Model file for the job. Use its own axes, mm. Coordinates: 2 decimals unless noted, no trailing zeros. Use CSV: the item, a comma, the result in double quotes. Start each with the question number.
(1) Cut at A-A on y = 1.25. Give the number of separate pieces and of enclosed holes in the cut face, plus the area to 3 significant figures.
(2) Probe L1, parallel to X at y = 1.95, z = 139.7; L2, parallel to X at y = 2.3, z = 19 (3 decimals); L3, parallel to Z at x = 38.5, y = 1.1. List the from-to ranges inside material, lowest first.
(3) Pin check, flat tip, straight feed: pin 1 Ø3 at (x, z) = (21.01, -39.81) entering from +Y. Stop position of the tip, or through.
```python
from build123d import *

# Parameters (mm, degrees)
PLATE_THICKNESS_DEPTH        = 3.175
SKETCH3_R                    = 2.159
MOUNTING_HOLES_DEPTH         = 159.781746826
SKETCH4_R                    = 1.905
JETSON_HOLES_W_O_MOUNT_DEPTH = 159.781746826
SKETCH5_R                    = 1.905
PDB_HOLES_DEPTH              = 159.781746826
SKETCH7_R                    = 1.27
PIXHAWK_HOLES_DEPTH          = 159.781746826
BATTERY_HOLES_DEPTH          = 159.781746826
SKETCH9_R                    = 2
CUT_EXTRUDE1_DEPTH           = 159.781746826
VENTRAL_CAMERA_HOLES_REACH   = 160.782
SKETCH10_R                   = 1


with BuildPart() as part:
    # Sketch2 → Plate Thickness (new body)
    with BuildSketch(Plane(origin=(0, 0, 0), x_dir=(1, 0, 0), z_dir=(0, 1, 0))):
        with BuildLine():
            Line((-41.275, 152.4), (41.275, 152.4))
            ThreePointArc((41.275, 152.4), (43.52006403, 151.47006403), (44.45, 149.225))
            Line((44.45, 149.225), (44.45, -149.225))
            ThreePointArc((44.45, -149.225), (43.52006403, -151.47006403), (41.275, -152.4))
            Line((41.275, -152.4), (-41.275, -152.4))
            ThreePointArc((-41.275, -152.4), (-43.52006403, -151.47006403), (-44.45, -149.225))
            Line((-44.45, -149.225), (-44.45, 149.225))
            ThreePointArc((-44.45, 149.225), (-43.52006403, 151.47006403), (-41.275, 152.4))
        make_face()
    extrude(amount=PLATE_THICKNESS_DEPTH)

    # Sketch3 → Mounting holes (cut, through all)
    with BuildSketch(Plane(origin=(0, 3.175, 0), x_dir=(1, 0, 0), z_dir=(0, 1, 0))):
        with Locations(Location((-38.1, 139.7, 0), (0, 0, 270))):
            Circle(SKETCH3_R)
        with Locations(Location((-38.1, 46.566666666, 0), (0, 0, 270))):
            Circle(SKETCH3_R)
        with Locations(Location((-38.1, -46.56666582, 0), (0, 0, 90))):
            Circle(SKETCH3_R)
        with Locations(Location((-38.1, -139.7, 0), (0, 0, 90))):
            Circle(SKETCH3_R)
        with Locations(Location((38.1, -139.7, 0), (0, 0, 270))):
            Circle(SKETCH3_R)
        with Locations(Location((38.1, -46.56666582, 0), (0, 0, 270))):
            Circle(SKETCH3_R)
        with Locations(Location((38.1, 46.566666666, 0), (0, 0, 90))):
            Circle(SKETCH3_R)
        with Locations(Location((38.1, 139.7, 0), (0, 0, 90))):
            Circle(SKETCH3_R)
        with Locations(Location((0, 139.7, 0), (0, 0, 270))):
            Circle(SKETCH3_R)
        with Locations(Location((0, -139.7, 0), (0, 0, 90))):
            Circle(SKETCH3_R)
    extrude(amount=-MOUNTING_HOLES_DEPTH, mode=Mode.SUBTRACT)

    # Sketch4 → Jetson Holes (w/o mount) (cut, through all)
    with BuildSketch(Plane(origin=(0, 3.175, 0), x_dir=(1, 0, 0), z_dir=(0, 1, 0))):
        with Locations(Location((-21.0058, 118.808268359, 0), (0, 0, 270))):
            Circle(SKETCH4_R)
        with Locations(Location((-21.0058, 39.814268359, 0), (0, 0, 270))):
            Circle(SKETCH4_R)
        with Locations(Location((21.0058, 39.814268359, 0), (0, 0, 90))):
            Circle(SKETCH4_R)
        with Locations(Location((21.0058, 118.808268359, 0), (0, 0, 90))):
            Circle(SKETCH4_R)
    extrude(amount=-JETSON_HOLES_W_O_MOUNT_DEPTH, mode=Mode.SUBTRACT)

    # Sketch5 → PDB holes (cut, through all)
    with BuildSketch(Plane(origin=(0, 3.175, 0), x_dir=(1, 0, 0), z_dir=(0, 1, 0))):
        with Locations(Location((-15.378405846, 116.28393812, 0), (0, 0, 270))):
            Circle(SKETCH5_R)
        with Locations(Location((14.618994154, 116.28393812, 0), (0, 0, 270))):
            Circle(SKETCH5_R)
        with Locations(Location((14.618994154, 86.28653812, 0), (0, 0, 270))):
            Circle(SKETCH5_R)
        with Locations(Location((-15.378405846, 86.28653812, 0), (0, 0, 270))):
            Circle(SKETCH5_R)
    extrude(amount=-PDB_HOLES_DEPTH, mode=Mode.SUBTRACT)

    # Sketch7 → PixHawk Holes (cut, through all)
    with BuildSketch(Plane(origin=(0, 3.175, 0), x_dir=(1, 0, 0), z_dir=(0, 1, 0))):
        with Locations(Location((-17.145, 14.489268954, 0), (0, 0, 270))):
            Circle(SKETCH7_R)
        with Locations(Location((-17.145, -70.600731046, 0), (0, 0, 270))):
            Circle(SKETCH7_R)
        with Locations(Location((17.145, -70.600731046, 0), (0, 0, 270))):
            Circle(SKETCH7_R)
        with Locations(Location((17.145, 14.489268954, 0), (0, 0, 270))):
            Circle(SKETCH7_R)
    extrude(amount=-PIXHAWK_HOLES_DEPTH, mode=Mode.SUBTRACT)

    # Sketch8 → Battery Holes (cut, through all)
    with BuildSketch(Plane(origin=(0, 3.175, 0), x_dir=(1, 0, 0), z_dir=(0, 1, 0))):
        with BuildLine():
            Line((-23.495, -0.005964701), (-23.495, -50.805964701))
            ThreePointArc((-23.495, -50.805964701), (-26.035, -53.345964701), (-28.575, -50.805964701))
            Line((-28.575, -50.805964701), (-28.575, -0.005964701))
            ThreePointArc((-28.575, -0.005964701), (-26.035, 2.534035299), (-23.495, -0.005964701))
        make_face()
        with BuildLine():
            Line((23.495, -0.005964701), (23.495, -50.805964701))
            ThreePointArc((23.495, -50.805964701), (26.035, -53.345964701), (28.575, -50.805964701))
            Line((28.575, -50.805964701), (28.575, -0.005964701))
            ThreePointArc((28.575, -0.005964701), (26.035, 2.534035299), (23.495, -0.005964701))
        make_face()
    extrude(amount=-BATTERY_HOLES_DEPTH, mode=Mode.SUBTRACT)

    # Sketch9 → Cut-Extrude1 (cut, through all)
    with BuildSketch(Plane(origin=(0, 3.175, 0), x_dir=(1, 0, 0), z_dir=(0, 1, 0))):
        with Locations(Location((6.833401633, -85.3, 0), (0, 0, 270))):
            Circle(SKETCH9_R)
        with Locations(Location((34.333401633, -85.3, 0), (0, 0, 270))):
            Circle(SKETCH9_R)
        with Locations(Location((34.333401633, -114.3, 0), (0, 0, 270))):
            Circle(SKETCH9_R)
        with Locations(Location((6.833401633, -114.3, 0), (0, 0, 270))):
            Circle(SKETCH9_R)
    extrude(amount=-CUT_EXTRUDE1_DEPTH, mode=Mode.SUBTRACT)

    # Sketch10 → Ventral Camera holes (cut, up to next)
    with BuildSketch(Plane(origin=(0, 3.175, 0), x_dir=(1, 0, 0), z_dir=(0, 1, 0)), mode=Mode.PRIVATE) as ventral_camera_holes_sk1:
        with Locations(Location((-38.125460092, -87.008641581, 0), (0, 0, 270))):
            Circle(SKETCH10_R)
    ventral_camera_holes_tool1 = extrude(ventral_camera_holes_sk1.sketch, amount=-VENTRAL_CAMERA_HOLES_REACH, mode=Mode.PRIVATE) & part.part
    # Sketch10 → Ventral Camera holes (cut, up to next)
    with BuildSketch(Plane(origin=(0, 3.175, 0), x_dir=(1, 0, 0), z_dir=(0, 1, 0)), mode=Mode.PRIVATE) as ventral_camera_holes_sk2:
        with Locations(Location((-38.1, -115.008630005, 0), (0, 0, 270))):
            Circle(SKETCH10_R)
    ventral_camera_holes_tool2 = extrude(ventral_camera_holes_sk2.sketch, amount=-VENTRAL_CAMERA_HOLES_REACH, mode=Mode.PRIVATE) & part.part
    # Sketch10 → Ventral Camera holes (cut, up to next)
    with BuildSketch(Plane(origin=(0, 3.175, 0), x_dir=(1, 0, 0), z_dir=(0, 1, 0)), mode=Mode.PRIVATE) as ventral_camera_holes_sk3:
        with Locations(Location((-10.126568972, -85.789139736, 0), (0, 0, 270))):
            Circle(SKETCH10_R)
    ventral_camera_holes_tool3 = extrude(ventral_camera_holes_sk3.sketch, amount=-VENTRAL_CAMERA_HOLES_REACH, mode=Mode.PRIVATE) & part.part
    # Sketch10 → Ventral Camera holes (cut, up to next)
    with BuildSketch(Plane(origin=(0, 3.175, 0), x_dir=(1, 0, 0), z_dir=(0, 1, 0)), mode=Mode.PRIVATE) as ventral_camera_holes_sk4:
        with Locations(Location((-10.126568972, -113.789139736, 0), (0, 0, 270))):
            Circle(SKETCH10_R)
    ventral_camera_holes_tool4 = extrude(ventral_camera_holes_sk4.sketch, amount=-VENTRAL_CAMERA_HOLES_REACH, mode=Mode.PRIVATE) & part.part
    add(ventral_camera_holes_tool1.solids().sort_by_distance((-38.12546, 3.175, 87.008642))[0], mode=Mode.SUBTRACT)
    add(ventral_camera_holes_tool2.solids().sort_by_distance((-38.1, 3.175, 115.00863))[0], mode=Mode.SUBTRACT)
    add(ventral_camera_holes_tool3.solids().sort_by_distance((-10.126569, 3.175, 85.78914))[0], mode=Mode.SUBTRACT)
    add(ventral_camera_holes_tool4.solids().sort_by_distance((-10.126569, 3.175, 113.78914))[0], mode=Mode.SUBTRACT)


solid = part.part
```
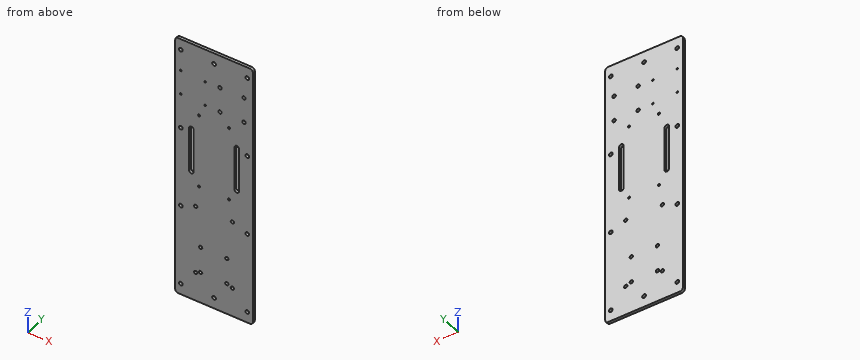
Outcome:
1,separate pieces,"1"
1,enclosed holes,"32"
1,area,"26,200 mm2"
2,L1,"-44.45 to -40.26, -35.94 to -2.16, 2.16 to 35.94, 40.26 to 44.45"
2,L2,"-44.45 to -28.575, -23.495 to 23.495, 28.575 to 44.45"
2,L3,"-152.4 to -141.82, -137.58 to -48.69, -44.45 to 44.45, 48.69 to 137.58, 141.82 to 152.4"
3,pin 1,"through"
